```python
from build123d import *

# Parameters (mm, degrees)
EXTRUDE_1_DEPTH           = 41
SKETCH_3_R                = 17
SKETCH_3_R_2              = 9
EXTRUDE_3_DEPTH           = 5
CUT_EXTRUDE_START         = -76
SKETCH_6_R                = 9
CUT_EXTRUDE_1_DEPTH       = 76
EXTRUDE_START             = 5
SKETCH_7_R                = 17
SKETCH_7_R_2              = 9
EXTRUDE_4_DEPTH           = 5
HOLE_WIZARD_M6_1_D        = 5
HOLE_WIZARD_M6_1_DEPTH    = 17
HOLE_WIZARD_M6_1_TIP      = 1.502151548
HOLE_WIZARD_5_0_5_1_D     = 5
HOLE_WIZARD_5_0_5_1_DEPTH = 5
HOLE_WIZARD_5_0_5_1_TIP   = 1.502151548
HOLE_WIZARD_M6_2_D        = 5
HOLE_WIZARD_M6_2_DEPTH    = 17
HOLE_WIZARD_M6_2_TIP      = 1.502151548
HOLE_WIZARD_5_0_5_2_D     = 5
HOLE_WIZARD_5_0_5_2_DEPTH = 17
HOLE_WIZARD_5_0_5_2_TIP   = 1.502151548


with BuildPart() as part:
    # 草图1 → 凸台-拉伸1 (new body)
    with BuildSketch(Plane.XY):
        with BuildLine():
            Line((38, 16.731473276), (38, -17.268526724))
            ThreePointArc((38, -17.268526724), (0, -55.268526724), (-38, -17.268526724))
            Line((-38, -17.268526724), (-38, 16.731473276))
            ThreePointArc((-38, 16.731473276), (0, 54.731473276), (38, 16.731473276))
        make_face()
        with BuildLine():
            Line((-19.73064692, 7), (-26.73064692, 7))
            Line((-26.73064692, 7), (-26.45655054, -7))
            Line((-26.45655054, -7), (-19.45655054, -7))
            ThreePointArc((-19.45655054, -7), (0, -39.268526724), (19.45655054, -7))
            Line((19.45655054, -7), (26.45655054, -7))
            Line((26.45655054, -7), (26.73064692, 7))
            Line((26.73064692, 7), (19.73064692, 7))
            ThreePointArc((19.73064692, 7), (0, 38.731473276), (-19.73064692, 7))
        make_face(mode=Mode.SUBTRACT)
    extrude(amount=EXTRUDE_1_DEPTH)

    # 草图3 → 凸台-拉伸3 (add)
    with BuildSketch(Plane.ZY.offset(38)):
        with Locations(Location((20.5, -0.04055331, 0), (0, 0, 99.3938106))):
            Circle(SKETCH_3_R)
        with Locations((20.5, -0.04055331)):
            Circle(SKETCH_3_R_2, mode=Mode.SUBTRACT)
    extrude(amount=EXTRUDE_3_DEPTH)

    # 草图6 → 切除-拉伸1 (cut)
    with BuildSketch(Plane.ZY.offset(38).offset(CUT_EXTRUDE_START)):
        with Locations(Location((20.5, -0.04055331, 0), (0, 0, 230.648614593))):
            Circle(SKETCH_6_R)
    extrude(amount=CUT_EXTRUDE_1_DEPTH, mode=Mode.SUBTRACT)

    # 草图7 → 凸台-拉伸4 (add)
    with BuildSketch(Plane(origin=(38, 0, 0), x_dir=(0, 0, -1), z_dir=(1, 0, 0)).offset(EXTRUDE_START)):
        with Locations(Location((-20.5, -0.04055331, 0), (0, 0, 80.6061894))):
            Circle(SKETCH_7_R)
        with Locations(Location((-20.5, -0.04055331, 0), (0, 0, 309.351385407))):
            Circle(SKETCH_7_R_2, mode=Mode.SUBTRACT)
    extrude(amount=-EXTRUDE_4_DEPTH)

    # M6 螺纹孔1
    with Locations(Plane(origin=(0, 47.027832747, 0), x_dir=(-1, 0, 0), z_dir=(0, 0, -1))):
        with Locations((0, 0), (-25.980762114, -15.296359471), (-28.977774789, -72.060930824), (0, -94.296359471), (28.977774789, -72.060930824), (25.980762114, -15.296359471)):
            Hole(HOLE_WIZARD_M6_1_D / 2, depth=HOLE_WIZARD_M6_1_DEPTH)
            with Locations((0, 0, -(HOLE_WIZARD_M6_1_DEPTH + HOLE_WIZARD_M6_1_TIP / 2))):  # 118° drill point
                Cone(0, HOLE_WIZARD_M6_1_D / 2, HOLE_WIZARD_M6_1_TIP, mode=Mode.SUBTRACT)

    # Ø5.0 (5) 直径孔1
    with Locations(Plane(origin=(15, 42.71223539, 0), x_dir=(-1, 0, 0), z_dir=(0, 0, -1))):
        with Locations((0, 0), (30, -85.961524227)):
            Hole(HOLE_WIZARD_5_0_5_1_D / 2, depth=HOLE_WIZARD_5_0_5_1_DEPTH)
            with Locations((0, 0, -(HOLE_WIZARD_5_0_5_1_DEPTH + HOLE_WIZARD_5_0_5_1_TIP / 2))):  # 118° drill point
                Cone(0, HOLE_WIZARD_5_0_5_1_D / 2, HOLE_WIZARD_5_0_5_1_TIP, mode=Mode.SUBTRACT)

    # M6 螺纹孔2
    with Locations(Plane(origin=(0, 46.731473276, 41), x_dir=(1, 0, 0), z_dir=(0, 0, 1))):
        with Locations((0, 0), (-25.980762114, -15), (25.980762114, -15), (30, -64), (-30, -64), (-15, -89.980762113), (15, -89.980762113)):
            Hole(HOLE_WIZARD_M6_2_D / 2, depth=HOLE_WIZARD_M6_2_DEPTH)
            with Locations((0, 0, -(HOLE_WIZARD_M6_2_DEPTH + HOLE_WIZARD_M6_2_TIP / 2))):  # 118° drill point
                Cone(0, HOLE_WIZARD_M6_2_D / 2, HOLE_WIZARD_M6_2_TIP, mode=Mode.SUBTRACT)

    # Ø5.0 (5) 直径孔2
    with Locations(Plane(origin=(-15, 42.71223539, 41), x_dir=(1, 0, 0), z_dir=(0, 0, 1))):
        with Locations((0, 0), (40.980762114, -74.980762114)):
            Hole(HOLE_WIZARD_5_0_5_2_D / 2, depth=HOLE_WIZARD_5_0_5_2_DEPTH)
            with Locations((0, 0, -(HOLE_WIZARD_5_0_5_2_DEPTH + HOLE_WIZARD_5_0_5_2_TIP / 2))):  # 118° drill point
                Cone(0, HOLE_WIZARD_5_0_5_2_D / 2, HOLE_WIZARD_5_0_5_2_TIP, mode=Mode.SUBTRACT)


solid = part.part
```
CAD build for the part. Positions are in the model's coordinates, mm. A direction names the side the tool comes from. Coordinates: 2 decimals unless noted, no trailing zeros. Order: outer loops, then holes, each group sorted by start corner. A loop starts at its lowest first (then second) coordinate and runs counter-clockwise, first axis right, second up. Notation, with made-up numbers: (17.5, 49) -> (29.5, 49) arc R19 ccw to (29.5, 63) -> close; hole circle Ø6 at (83.5, -35). An arc over 180 degrees is marked (long way). Use one line per item in the form item = value. Start each with the question number.
1) Tool access for faces 5 (the cylindrical face through (1.34, -45.16, 8.62)), 6 (the flat face through (-38, -16, 29)), 7 (the flat face through (-23, -7, 33)), 8 (the cylindrical face through (-14.46, 40.27, 32.38)): list every direction of +Z, -Z, +X, -X, +Y, -Y with a clear straight run to the whole face (end or side of a thin tool).
2) Band-saw the part on D-D on y = 14. Give the cut face in (x, z).
3) Drill centre lines: L1, parallel to X at y = 32, z = 14; L2, parallel to Y at x = 32, z = 33; L3, parallel to X at y = 0, z = 31.5. Where is each one in solid material? Low to high. Write a range as [from, to].
4) Drop flat-ended pins along their axis: pin 1 (2 mm diameter, centred on x = 22.5, z = 11, fed in from -Y); pin 2 (2 mm diameter, centred on x = 24, z = 36, fed in from +Y); pin 3 (7.5 mm diameter, centred on x = -22, z = 30.5, fed in from +Y); pin 4 (16 mm diameter, centred on y = -0.04, z = 20.5, fed in from +X). Give the stop position or say it passes through.
5) Pull direction Y, two halves, no side cores. Call faces 1 (the cylindrical face through (0.84, -55.26, 20.21)), 2 (the cylindrical face through (27.325, 33.839, 8.619)), 3 (the cylindrical face through (26.99, -26.55, 8.62)), 4 (the flat face through (26, 13, 0)): +Y half, -Y half, draft (parallel to the pull), parting line (faces both ways), or undercut.
6) Band-saw the part on B-B on x = 4.5. Give the cut face in (y, z).
7) Band-saw the part on A-A on y = 26. Give the cut face in (x, z).
Entries:
q1.face_5 = -Z
q1.face_6 = -X
q1.face_7 = +Z, -Z
q1.face_8 = +Z
q2.outline = (-43, 10.92) -> (-38, 10.92) -> (-38, 0) -> (-21.83, 0) -> (-21.83, 41) -> (-38, 41) -> (-38, 30.08) -> (-43, 30.08) -> close; (21.83, 0) -> (38, 0) -> (38, 10.92) -> (43, 10.92) -> (43, 30.08) -> (38, 30.08) -> (38, 41) -> (21.83, 41) -> close
q3.L1 = [-34.8, -28.47], [-23.5, -15.84], [15.84, 23.5], [28.47, 34.8]
q3.L2 = [-37.76, -18.77], [-15.77, 37.23]
q3.L3 = [-43, -26.59], [26.59, 43]
q4.pin_1 = -48.6
q4.pin_2 = 46.98
q4.pin_3 = 50.06
q4.pin_4 = through
q5.face_1 = -Y half
q5.face_2 = undercut
q5.face_3 = undercut
q5.face_4 = draft
q6.outline = (-55, 0) -> (-38.8, 0) -> (-38.8, 41) -> (-55, 41) -> close; (38.27, 0) -> (54.46, 0) -> (54.46, 41) -> (38.27, 41) -> close
q7.outline = (-36.85, 0) -> (-19.95, 0) -> (-19.95, 41) -> (-36.85, 41) -> close; (19.95, 0) -> (36.85, 0) -> (36.85, 41) -> (19.95, 41) -> close
